Geometry: final body of the model. Coordinates: model frame, mm. A direction names the side the tool comes from. Round coordinates to 2 decimals unless told otherwise and drop trailing zeros. Loops run counter-clockwise (first coordinate to the right, second up) from the corner with the lowest first, then second, coordinate; pieces in that order, holes last. Notation, with made-up numbers: (-6, -6.75) - (31, -6.75) arc R35 ccw to (31, 28.25) - close; hole circle Ø3 at (-19.5, -27). An arc over 180 degrees is marked (long way). Use CSV: the item, a comma, the result in double quotes.
from build123d import *

# Parameters (mm, degrees)
BOSS_EXTRUDE1_DEPTH = 5
SKETCH2_W           = 5.125
SKETCH2_H           = 17.5
CUT_EXTRUDE1_DEPTH  = 5


with BuildPart() as part:
    # Sketch1 → Boss-Extrude1 (new body)
    with BuildSketch(Plane.XY):
        with BuildLine():
            Line((2, 0), (68, 0))
            ThreePointArc((68, 0), (69.414213562, 0.585786438), (70, 2))
            Line((70, 2), (70, 48))
            ThreePointArc((70, 48), (69.414213562, 49.414213562), (68, 50))
            Line((68, 50), (2, 50))
            ThreePointArc((2, 50), (0.585786438, 49.414213562), (0, 48))
            Line((0, 48), (0, 2))
            ThreePointArc((0, 2), (0.585786438, 0.585786438), (2, 0))
        make_face()
    extrude(amount=BOSS_EXTRUDE1_DEPTH)

    # Sketch2 → Cut-Extrude1 (cut)
    with BuildSketch(Plane(origin=(-23.39926368, 94.916866164, 5), x_dir=(1, 0, 0), z_dir=(0, 0, 1))):
        with Locations((39.316333928, -53.666866164)):
            Rectangle(SKETCH2_W, SKETCH2_H)
        with Locations((77.482193432, -53.666866164)):
            Rectangle(SKETCH2_W, SKETCH2_H)
        with Locations((39.316333928, -86.166866164)):
            Rectangle(SKETCH2_W, SKETCH2_H)
        with Locations((77.482193432, -86.166866164)):
            Rectangle(SKETCH2_W, SKETCH2_H)
    extrude(amount=-CUT_EXTRUDE1_DEPTH, mode=Mode.SUBTRACT)


solid = part.part
Item 1: Section B-B on z = 2.3. Return the cut outline in (x, y), plus the area to 3 significant figures.
Final values:
outline,"(0, 2) arc R2 ccw to (2, 0) - (13.35, 0) - (13.35, 17.5) - (18.48, 17.5) - (18.48, 0) - (51.52, 0) - (51.52, 17.5) - (56.65, 17.5) - (56.65, 0) - (68, 0) arc R2 ccw to (70, 2) - (70, 48) arc R2 ccw to (68, 50) - (56.65, 50) - (56.65, 32.5) - (51.52, 32.5) - (51.52, 50) - (18.48, 50) - (18.48, 32.5) - (13.35, 32.5) - (13.35, 50) - (2, 50) arc R2 ccw to (0, 48) - close"
area,"3,140 mm²"
Item 2: Mould query, pull axis X, two halves, no side actions, for faces 4 (the flat face through (8, 50, 2)), 5 (the flat face through (13.355, 9, 3)), 6 (the cylindrical face through (0.6, 49.43, 2.46)). Classes: released by +X, released by -X, zero draft, split by the parting line, or undercut.
Final values:
face 4,"zero draft"
face 5,"undercut"
face 6,"released by -X"
Item 3: Pin query (flat end, axial travel): P1, Ø1, axis at x = 44.5, z = 4, coming from the -Y side; P2, Ø2.5, axis at x = 54, z = 3.5, coming from the -Y side. Return the tip coordinate at first contact, or that it passes through.
Final values:
P1,"stops at y = 0"
P2,"stops at y = 17.5"
Item 4: Section A-A on y = 6. Return the cut outline in (x, z).
Final values:
outline,"(0, 0) - (13.35, 0) - (13.35, 5) - (0, 5) - close; (18.48, 0) - (51.52, 0) - (51.52, 5) - (18.48, 5) - close; (56.65, 0) - (70, 0) - (70, 5) - (56.65, 5) - close"
Item 5: Material intervals for line 1 (X direction, y = 47.5, z = 1), sorted ascending.
Final values:
line 1,"x = 0 to 13.35, 18.48 to 51.52, 56.65 to 70"
Item 6: Reachability of faces 1 (the flat face through (8, 0, 2)), 2 (the flat face through (16, 17.5, 3)), 3 (the flat face through (13.355, 41, 3)) from +Z, -Z, +X, -X, +Y, -Y: full face, straight path, thin tool, end or side. Return the list, or none.
Final values:
face 1,"+Z, -Z, +X, -X, -Y"
face 2,"+Z, -Z, -Y"
face 3,"+Z, -Z, +Y"
